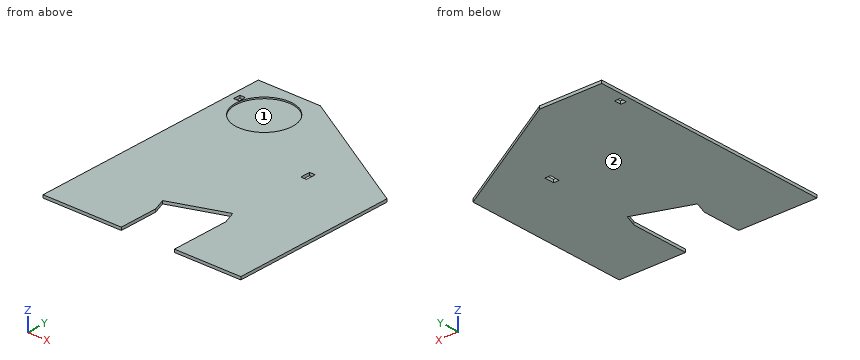
```python
from build123d import *

# Parameters (mm, degrees)
BOSS_EXTRUDE1_DEPTH = 2
SKETCH3_W           = 4.004504799
SKETCH3_H           = 7.007808652
SKETCH3_W_2         = 4
SKETCH3_H_2         = 5
CUT_EXTRUDE1_DEPTH  = 10
SKETCH4_R           = 20
CUT_EXTRUDE2_DEPTH  = 1


with BuildPart() as part:
    # Sketch1 → Boss-Extrude1 (new body)
    with BuildSketch(Plane.XY):
        Polygon((-70, 100), (-70, -72.799540117), (70, -72.799540117), (70, 44.524791386), (-26.08587988, 100), align=None)
    extrude(amount=BOSS_EXTRUDE1_DEPTH)

    # Sketch3 → Cut-Extrude1 (cut)
    with BuildSketch(Plane.XY.offset(2)):
        with Locations((21.429491924, 36.193920339)):
            Rectangle(SKETCH3_W, SKETCH3_H)
        with Locations((-64, 78.155444566)):
            Rectangle(SKETCH3_W_2, SKETCH3_H_2)
        Polygon((-14.572335871, -75.184527756), (23.015368961, -75.184527756), (23.015368961, -31.503722023), (19.595167527, -22.106795815), (-17.992537304, -35.787601548), (-14.572335871, -45.184527756), align=None)
    extrude(amount=-CUT_EXTRUDE1_DEPTH, mode=Mode.SUBTRACT)

    # Sketch4 → Cut-Extrude2 (cut)
    with BuildSketch(Plane.XY.offset(2)):
        with Locations((-41.723720558, 72.655444566)):
            Circle(SKETCH4_R)
    extrude(amount=-CUT_EXTRUDE2_DEPTH, mode=Mode.SUBTRACT)


solid = part.part
```
For this review, take the finished solid that the model builds, in its own axes (mm). Face numbers are marked on the shaded views. Round coordinates to 2 decimals unless told otherwise and drop trailing zeros. Write each loop counter-clockwise with the first axis right and the second up, starting at its lowest first coordinate (ties: lowest second). Pieces come first, ordered by that corner, then holes.
1) Mouldability with a two-part tool opening along Y and no side actions: class the marked faces 1 and 2 as +Y half, -Y half, draft (parallel to the pull), parting line (faces both ways), or undercut.
Answer below:
face 1: undercut
face 2: draft
2) Take a section at C-C on y = 65.5. Give the boundary of the cut face in (x, z), then the cut area to 3 significant figures.
Answer below:
outline: (-70, 0) - (33.67, 0) - (33.67, 2) - (-23.05, 2) - (-23.05, 1) - (-60.4, 1) - (-60.4, 2) - (-70, 2) - close
area: 170 mm2
3) Take a section at D-D on x = 50.5. Give the boundary of the cut face in (y, z).
Answer below:
outline: (-72.8, 0) - (55.78, 0) - (55.78, 2) - (-72.8, 2) - close
4) Take a section at B-B on x = -30.5. Give the boundary of the cut face in (y, z).
Answer below:
outline: (-72.8, 0) - (100, 0) - (100, 2) - (89.21, 2) - (89.21, 1) - (56.1, 1) - (56.1, 2) - (-72.8, 2) - close
5) Take a section at A-A on z = 0.4. Give the boundary of the cut face in (x, y), then the cut area to 3 significant figures.
Answer below:
outline: (-70, -72.8) - (-14.57, -72.8) - (-14.57, -45.18) - (-17.99, -35.79) - (19.6, -22.11) - (23.02, -31.5) - (23.02, -72.8) - (70, -72.8) - (70, 44.52) - (-26.09, 100) - (-70, 100) - close; hole (-66, 75.66) - (-62, 75.66) - (-62, 80.66) - (-66, 80.66) - close; hole (19.43, 32.69) - (23.43, 32.69) - (23.43, 39.7) - (19.43, 39.7) - close
area: 19,800 mm2
6) Insertion check: pin 1 Ø2 at (x, y) = (20, -24) entering from +Z; pin 2 Ø1 at (x, z) = (22.5, 1) entering from +Y. Each pin has a flat end and moves straight along its axis. Give the tip position at first contact, or say it passes through.
Answer below:
pin 1: stops at z = 2
pin 2: stops at y = 72.24
7) For line 1 along Y through (x, z) = (-41, 1.6); line 2 along X through (y, z) = (-50.5, 1.85); line 3 along Y through (x, z) = (-55, 1.05), list the stretches that pass through material, from the lowest coordinate up.
Answer below:
line 1: y = -72.8 to 52.67, 92.64 to 100
line 2: x = -70 to -14.57, 23.02 to 70
line 3: y = -72.8 to 57.7, 87.61 to 100
